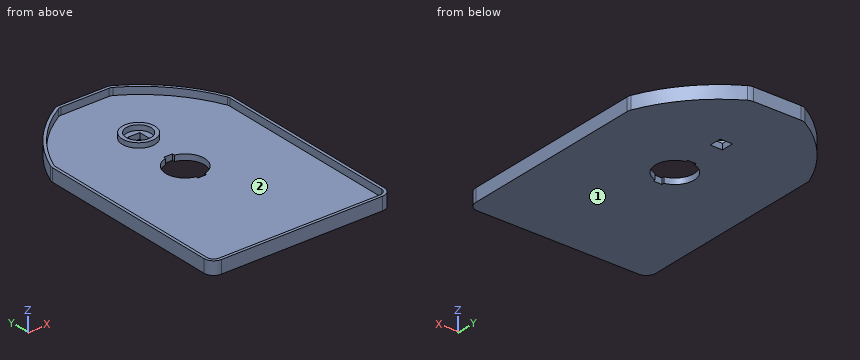
from build123d import *

# Parameters (mm, degrees)
BOSS_EXTRUDE1_DEPTH = 2.4
EXTRUDE_THIN1_DEPTH = 3
SKETCH3_R           = 8.05
CUT_EXTRUDE1_DEPTH  = 71.680761173
SKETCH4_R           = 5.2
SKETCH4_R_2         = 5
CUT_EXTRUDE2_DEPTH  = 0.8
SKETCH5_W           = 5.1
SKETCH5_H           = 5.1
SKETCH5_W_2         = 4.8
SKETCH5_H_2         = 4.8
CUT_EXTRUDE5_DEPTH  = 71.823230652
BOSS_EXTRUDE2_START = 2
SKETCH8_R           = 6.8
SKETCH8_R_2         = 5.2
BOSS_EXTRUDE2_DEPTH = 2


with BuildPart() as part:
    # Sketch1 → Boss-Extrude1 (new body)
    with BuildSketch(Plane.XY):
        with BuildLine():
            Line((37.4, -55.9), (37.4, 21.822390499))
            ThreePointArc((37.4, 21.822390499), (37.321949444, 22.608719027), (37.090843722, 23.364360867))
            ThreePointArc((37.090843722, 23.364360867), (26.864407476, 39.766080063), (11.953879914, 52.065371047))
            ThreePointArc((11.953879914, 52.065371047), (10.982508971, 52.471443007), (9.938833779, 52.61))
            Line((9.938833779, 52.61), (-9.938833779, 52.61))
            ThreePointArc((-9.938833779, 52.61), (-10.982508971, 52.471443007), (-11.953879914, 52.065371047))
            ThreePointArc((-11.953879914, 52.065371047), (-26.864407476, 39.766080063), (-37.090843722, 23.364360867))
            ThreePointArc((-37.090843722, 23.364360867), (-37.321949444, 22.608719027), (-37.4, 21.822390499))
            Line((-37.4, 21.822390499), (-37.4, -55.9))
            ThreePointArc((-37.4, -55.9), (-36.228427125, -58.728427125), (-33.4, -59.9))
            Line((-33.4, -59.9), (33.4, -59.9))
            ThreePointArc((33.4, -59.9), (36.228427125, -58.728427125), (37.4, -55.9))
        make_face()
    extrude(amount=BOSS_EXTRUDE1_DEPTH)

    # Sketch2 → Extrude-Thin1 (add)
    with BuildSketch(Plane.XY.offset(2.4)):
        with BuildLine():
            Line((37.4, -55.9), (37.4, 21.822390499))
            ThreePointArc((37.4, 21.822390499), (37.321949444, 22.608719027), (37.090843722, 23.364360867))
            ThreePointArc((37.090843722, 23.364360867), (26.864407476, 39.766080063), (11.953879914, 52.065371047))
            ThreePointArc((11.953879914, 52.065371047), (10.982508971, 52.471443007), (9.938833779, 52.61))
            Line((9.938833779, 52.61), (-9.938833779, 52.61))
            ThreePointArc((-9.938833779, 52.61), (-10.982508971, 52.471443007), (-11.953879914, 52.065371047))
            ThreePointArc((-11.953879914, 52.065371047), (-26.864407476, 39.766080063), (-37.090843722, 23.364360867))
            ThreePointArc((-37.090843722, 23.364360867), (-37.321949444, 22.608719027), (-37.4, 21.822390499))
            Line((-37.4, 21.822390499), (-37.4, -55.9))
            ThreePointArc((-37.4, -55.9), (-36.228427125, -58.728427125), (-33.4, -59.9))
            Line((-33.4, -59.9), (33.4, -59.9))
            ThreePointArc((33.4, -59.9), (36.228427125, -58.728427125), (37.4, -55.9))
        make_face()
        with BuildLine():
            Line((36.2, -55.9), (36.2, 21.822390499))
            ThreePointArc((36.2, 21.822390499), (36.145364611, 22.372820469), (35.983590606, 22.901769756))
            ThreePointArc((35.983590606, 22.901769756), (25.961683084, 38.975454569), (11.349366074, 51.028759733))
            ThreePointArc((11.349366074, 51.028759733), (10.669406413, 51.313010105), (9.938833779, 51.41))
            Line((9.938833779, 51.41), (-9.938833779, 51.41))
            ThreePointArc((-9.938833779, 51.41), (-10.669406413, 51.313010105), (-11.349366074, 51.028759733))
            ThreePointArc((-11.349366074, 51.028759733), (-25.961683084, 38.975454569), (-35.983590606, 22.901769756))
            ThreePointArc((-35.983590606, 22.901769756), (-36.145364611, 22.372820469), (-36.2, 21.822390499))
            Line((-36.2, 21.822390499), (-36.2, -55.9))
            ThreePointArc((-36.2, -55.9), (-35.379898987, -57.879898987), (-33.4, -58.7))
            Line((-33.4, -58.7), (33.4, -58.7))
            ThreePointArc((33.4, -58.7), (35.379898987, -57.879898987), (36.2, -55.9))
        make_face(mode=Mode.SUBTRACT)
    extrude(amount=EXTRUDE_THIN1_DEPTH)

    # Sketch3 → Cut-Extrude1 (cut, through all)
    with BuildSketch(Plane.XY.offset(2.4)):
        with BuildLine():
            Line((1.8, 8.8223931), (-1.8, 8.8223931))
            Line((-1.8, 8.8223931), (-1.8, 7.846177413))
            ThreePointArc((-1.8, 7.846177413), (0, 8.05), (1.8, 7.846177413))
            Line((1.8, 7.846177413), (1.8, 8.8223931))
        make_face()
        with BuildLine():
            ThreePointArc((1.8, -7.846177413), (0, -8.05), (-1.8, -7.846177413))
            Line((-1.8, -7.846177413), (-1.8, -8.8223931))
            Line((-1.8, -8.8223931), (1.8, -8.8223931))
            Line((1.8, -8.8223931), (1.8, -7.846177413))
        make_face()
        Circle(SKETCH3_R)
    extrude(amount=-CUT_EXTRUDE1_DEPTH, mode=Mode.SUBTRACT)

    # Sketch4 → Cut-Extrude2 (cut)
    with BuildSketch(Plane.XY.offset(2.4)):
        with Locations((0, 23.9)):
            Circle(SKETCH4_R)
        with Locations((0, 23.9)):
            Circle(SKETCH4_R_2, mode=Mode.SUBTRACT)
    extrude(amount=-CUT_EXTRUDE2_DEPTH, mode=Mode.SUBTRACT)

    # Sketch5 → Cut-Extrude5 (cut, through all)
    # profile 1 of 2: a face of its own
    with BuildSketch(Plane(origin=(0, 0, 0), x_dir=(-1, 0, 0), z_dir=(0, 0, -1))):
        with Locations((0, 23.9)):
            Rectangle(SKETCH5_W, SKETCH5_H)
        with Locations((0, 23.9)):
            Rectangle(SKETCH5_W_2, SKETCH5_H_2, mode=Mode.SUBTRACT)
    # profile 2 of 2: a face of its own
    with BuildSketch(Plane(origin=(0, 0, 0), x_dir=(-1, 0, 0), z_dir=(0, 0, -1))):
        with Locations((0, 23.9)):
            Rectangle(SKETCH5_W_2, SKETCH5_H_2)
    extrude(amount=-CUT_EXTRUDE5_DEPTH, mode=Mode.SUBTRACT)

    # Sketch8 → Boss-Extrude2 (add)
    with BuildSketch(Plane.XY.offset(2.4).offset(BOSS_EXTRUDE2_START)):
        with Locations((0, 23.9)):
            Circle(SKETCH8_R)
        with Locations((0, 23.9)):
            Circle(SKETCH8_R_2, mode=Mode.SUBTRACT)
    extrude(amount=-BOSS_EXTRUDE2_DEPTH)


solid = part.part
The model under review builds one solid part; all positions refer to its coordinate system, in mm. Face numbers are marked on the shaded views. Round coordinates to 2 decimals unless told otherwise and drop trailing zeros. Loops run counter-clockwise (first coordinate to the right, second up) from the corner with the lowest first, then second, coordinate; pieces in that order, holes last. Notation, with made-up numbers: M 22.5,1 L 36.5,1 A26 cw 36.5,34 Z; hole C -32,23 d6. An arc over 180 degrees is marked long. Answer as a JSON object with one key per item and string values.
Item 1: For line 1 along Y through (x, z) = (0, 3.05); line 2 along X through (y, z) = (-40.5, 4.2); line 3 along Y through (x, z) = (-2, 4.45), list the stretches that pass through material, from the lowest coordinate up.
Check sheet entries:
{"line 1": "-59.9 to -58.7, 17.1 to 18.7, 29.1 to 30.7, 51.41 to 52.61", "line 2": "-37.4 to -36.2, 36.2 to 37.4", "line 3": "-59.9 to -58.7, 51.41 to 52.61"}
Item 2: Clearance check with flat-ended pins moving along their axes: P1, Ø15, axis at x = -2.5, y = 20.5, coming from the +Z side; P2, Ø10, axis at x = 9, y = 33, coming from the +Z side; P3, Ø0.7, axis at y = 25, z = 1, coming from the +X side. State where each tip first meets the part, or that it passes through.
Check sheet entries:
{"P1": "z = 4.4", "P2": "z = 2.4", "P3": "x = 36.54"}
Item 3: We need section A-A, the plane x = 0. State the section outline as (y, z) points.
Check sheet entries:
{"outline": "M -59.9,0 L -8.82,0 L -8.82,2.4 L -58.7,2.4 L -58.7,5.4 L -59.9,5.4 Z; M 8.82,0 L 21.35,0 L 21.35,2.4 L 18.9,2.4 L 18.9,1.6 L 18.7,1.6 L 18.7,4.4 L 17.1,4.4 L 17.1,2.4 L 8.82,2.4 Z; M 26.45,0 L 52.61,0 L 52.61,5.4 L 51.41,5.4 L 51.41,2.4 L 30.7,2.4 L 30.7,4.4 L 29.1,4.4 L 29.1,1.6 L 28.9,1.6 L 28.9,2.4 L 26.45,2.4 Z"}
Item 4: We need section C-C, the plane x = -29.5. State the section outline as (y, z) points, and give its area (3 significant figures).
Check sheet entries:
{"outline": "M -59.9,0 L 36.54,0 L 36.54,5.4 L 34.52,5.4 L 34.52,2.4 L -58.7,2.4 L -58.7,5.4 L -59.9,5.4 Z", "area": "241 mm2"}
Item 5: The part is to be moulded in two halves that separate along X. For the marked faces 1 and 2, say which applies: +X half, -X half, draft (parallel to the pull), parting line (faces both ways), or undercut.
Check sheet entries:
{"face 1": "draft", "face 2": "undercut"}
Item 6: We need section B-B, the plane y = 4. State the section outline as (x, z) points.
Check sheet entries:
{"outline": "M -37.4,0 L -6.99,0 L -6.99,2.4 L -36.2,2.4 L -36.2,5.4 L -37.4,5.4 Z; M 6.99,0 L 37.4,0 L 37.4,5.4 L 36.2,5.4 L 36.2,2.4 L 6.99,2.4 Z"}
Item 7: We need section D-D, the plane y = 45.5. State the section outline as (x, z) points, and give its area (3 significant figures).
Check sheet entries:
{"outline": "M -21.11,0 L 21.11,0 L 21.11,5.4 L 19.26,5.4 L 19.26,2.4 L -19.26,2.4 L -19.26,5.4 L -21.11,5.4 Z", "area": "112 mm2"}
